Could you check a few things on this model? Use its own coordinates, in mm. A direction names the side the tool comes from. Round coordinates to 2 decimals unless told otherwise and drop trailing zeros. Write each loop counter-clockwise with the first axis right and the second up, starting at its lowest first coordinate (ties: lowest second). Pieces come first, ordered by that corner, then holes. Notation, with made-up numbers: (84.25, 20.5) -> (123.25, 20.5) arc R23 ccw to (123.25, 49.5) -> close; hole circle Ø3 at (68, -15.5). An arc over 180 degrees is marked (long way). Answer as CSV lines item,"result". Start each with the question number.
Q1. For faces 5 (the flat face through (-98.855, -3.131, 107.621)), 6 (the flat face through (-111, -6.35, 91)), which set-ups out of +Z, -Z, +X, -X, +Y, -Y let a thin tool reach every point of the face, with its end or its side?
Q2. Imagine slicing it at C-C on x = -25.4. Please give me the cut outline in (y, z), and give its area (3 significant figures).
Q3. Imagine slicing it at B-B on z = 203.2. Please give me the cut outline in (x, y).
Q4. Will these pins go through, and if not, where does the flat tip stop? pin 1 Ø11 at (x, z) = (-76.2, 203.2) entering from -Y; pin 2 Ø1.5 at (y, z) = (-5.5, 66) entering from -X; pin 3 Ø3 at (y, z) = (-3, 159) entering from +X; pin 4 Ø2 at (y, z) = (-3.5, 191) entering from -X.
Q5. If we mould it in two halves opening along Z, with no side actions, what happens to faces 1 (the flat face through (0, -3, 20)), 2 (the cylindrical face through (-53.97, -3.13, 20.78)), 3 (the cylindrical face through (-73.39, -3.13, 197.79)), 4 (the cylindrical face through (-75.747, -3.131, 228.596))? For each: pulls with the +Z half, pulls with the -Z half, needs draft (parallel to the pull), parting line crosses it, or undercut.
Q6. Imagine slicing it at A-A on x = -76.2. Give the number of separate pieces and of enclosed holes in the cut face, and give its area (3 significant figures).
Q7. If I drill on line 1 (Z direction, x = -76.2, y = -3.5) (1 decimal); line 2 (X direction, y = -2.75, z = 23); line 3 (X direction, y = -4.75, z = 196.5), over which ranges is the centre line in solid material (lowest first)? Write a range as [from, to].
from build123d import *

# Parameters (mm, degrees)
F0_R     = 10.795
F0_R_2   = 3.175
F0_R_3   = 6.096
F1_DEPTH = 6.35


with BuildPart() as f1:
    # F0 (on Front) → F1 (new body)
    with BuildSketch(Plane.XZ):
        with BuildLine():
            Line((-152.4, 0), (0, 0))
            Line((0, 0), (0, 41.275))
            Line((0, 41.275), (-51.915237, 210.64381))
            ThreePointArc((-51.915237, 210.64381), (-76.2, 228.6), (-100.484763, 210.64381))
            Line((-100.484763, 210.64381), (-152.4, 41.275))
            Line((-152.4, 41.275), (-152.4, 0))
        make_face()
        with Locations((-127, 20.6375)):
            Circle(F0_R, mode=Mode.SUBTRACT)
        with Locations((-101.6, 20.6375)):
            Circle(F0_R_2, mode=Mode.SUBTRACT)
        with Locations((-50.8, 20.6375)):
            Circle(F0_R_2, mode=Mode.SUBTRACT)
        with Locations((-25.4, 20.6375)):
            Circle(F0_R, mode=Mode.SUBTRACT)
        with BuildLine():
            Line((-37.502079, 41.275), (-114.897921, 41.275))
            ThreePointArc((-114.897921, 41.275), (-117.450849, 42.562361), (-117.933516, 45.380476))
            Line((-117.933516, 45.380476), (-79.235595, 171.628974))
            ThreePointArc((-79.235595, 171.628974), (-76.2, 173.873498), (-73.164405, 171.628974))
            Line((-73.164405, 171.628974), (-34.466484, 45.380476))
            ThreePointArc((-34.466484, 45.380476), (-34.949151, 42.562361), (-37.502079, 41.275))
        make_face(mode=Mode.SUBTRACT)
        with Locations((-76.2, 203.2)):
            Circle(F0_R_3, mode=Mode.SUBTRACT)
    extrude(amount=F1_DEPTH)


solid = f1.part
Checks:
1,face 5,"+Y, -Y"
1,face 6,"+Z, -Z, +X, -X, -Y"
2,outline,"(-6.35, 0) -> (0, 0) -> (0, 9.84) -> (-6.35, 9.84) -> close; (-6.35, 31.43) -> (0, 31.43) -> (0, 124.14) -> (-6.35, 124.14) -> close"
2,area,"651 mm^2"
3,outline,"(-102.77, -6.35) -> (-82.3, -6.35) -> (-82.3, 0) -> (-102.77, 0) -> close; (-70.1, -6.35) -> (-49.63, -6.35) -> (-49.63, 0) -> (-70.1, 0) -> close"
4,pin 1,"through"
4,pin 2,"x = -145.05"
4,pin 3,"x = -35.63"
4,pin 4,"x = -106.81"
5,face 1,"needs draft"
5,face 2,"undercut"
5,face 3,"undercut"
5,face 4,"pulls with the +Z half"
6,separate pieces,"3"
6,enclosed holes,"0"
6,area,"532 mm^2"
7,line 1,"[0, 41.3], [173.9, 197.1], [209.3, 228.6]"
7,line 2,"[-152.4, -137.53], [-116.47, -103.72], [-99.48, -52.92], [-48.68, -35.93], [-14.87, 0]"
7,line 3,"[-104.82, -47.58]"
